Source: CAD feature listing. Evaluate the final solid. Frame: model axes, mm. A direction names the side the tool comes from. Coordinates: 2 decimals unless noted, no trailing zeros. Order: outer loops, then holes, each group sorted by start corner. A loop starts at its lowest first (then second) coordinate and runs counter-clockwise, first axis right, second up.
Item 1: Section C-C on x = 4. Return the cut outline in (y, z), then the cut area to 3 significant figures.
Item 2: Reachability of faces 1 (the flat face through (80.5, 0, 8.2)), 2 (the flat face through (82.5, 0, 0)) from +Z, -Z, +X, -X, +Y, -Y: full face, straight path, thin tool, end or side. Return the list, or none.
Item 3: Section A-A on y = 0. Return the cut outline in (x, z).
Item 4: Ray query, line 1 (X direction, y = 0, z = -3.75); line 2 (X direction, y = -1.25, z = 9.25); line 3 (Y direction, x = 4, z = -5.25). Return the intervals inside material, ascending.
Item 5: Contact query for flat-ended pins moving along their axis: P1, Ø1, axis at x = 52.5, y = -2, coming from the +Z side; P2, Ø1, axis at x = 30.5, y = -6, coming from the +Z side; P3, Ø6, axis at x = 45.5, z = -3.5, coming from the +Y side; P4, Ø8, axis at y = 7, z = 7.5, coming from the -X side. Output: stop coordinate, or through.
Item 6: Section B-B on x = 60. Return the cut outline in (y, z), then the cut area to 3 significant figures.
from build123d import *

# Parameters (mm, degrees)
SCHNITT_LINEAR_AUSTRAGEN1_REACH             = 12
SKIZZE2_R                                   = 1
SCHNITT_LINEAR_AUSTRAGEN1_DIRECTION_2_DEPTH = 11
VERRUNDUNG1_R                               = 1


with BuildPart() as part:
    # Skizze1 → Rotation1 (revolve)
    with BuildSketch(Plane.XY):
        Polygon((0, 0), (0, 8), (80.5, 8), (80.5, 10), (82.5, 10), (82.5, 0), align=None)
    revolve(axis=Axis((-15.956588212, 0, 0), (1, 0, 0)))

    # Skizze2 → Schnitt-Linear austragen1 (cut, up to next)
    with BuildSketch(Plane.XY, mode=Mode.PRIVATE) as schnitt_linear_austragen1_sk1:
        with Locations((4, 0)):
            Circle(SKIZZE2_R)
    schnitt_linear_austragen1_tool1 = extrude(schnitt_linear_austragen1_sk1.sketch, amount=-SCHNITT_LINEAR_AUSTRAGEN1_REACH, mode=Mode.PRIVATE) & part.part
    add(schnitt_linear_austragen1_tool1.solids().sort_by_distance((4, 0, 0))[0], mode=Mode.SUBTRACT)

    # Skizze2 → Schnitt-Linear austragen1 direction 2 (cut)
    with BuildSketch(Plane.XY):
        with Locations((4, 0)):
            Circle(SKIZZE2_R)
    extrude(amount=SCHNITT_LINEAR_AUSTRAGEN1_DIRECTION_2_DEPTH, mode=Mode.SUBTRACT)

    # Verrundung1
    verrundung1_edges = [part.edges().sort_by_distance(p)[0] for p in [
        (0, -8, 0),
    ]]
    fillet(verrundung1_edges, radius=VERRUNDUNG1_R)


solid = part.part
Answer list:
1. outline: (-1, -7.94) - (-1, 7.94) arc R8 ccw to start; (1, -7.94) arc R8 ccw to (1, 7.94) - close
1. area: 169 mm2
2. face 1: -X
2. face 2: +Z, -Z, +X, +Y, -Y
3. outline: (0, -7) arc R1 ccw to (1, -8) - (3, -8) - (3, 8) - (1, 8) arc R1 ccw to (0, 7) - close; (5, -8) - (80.5, -8) - (80.5, -10) - (82.5, -10) - (82.5, 10) - (80.5, 10) - (80.5, 8) - (5, 8) - close
4. line 1: x = 0 to 3, 5 to 82.5
4. line 2: x = 80.5 to 82.5
4. line 3: y = -6.04 to -1, 1 to 6.04
5. P1: stops at z = 7.86
5. P2: stops at z = 5.81
5. P3: stops at y = 7.98
5. P4: stops at x = 0
6. outline: circle Ø16 at (0, 0)
6. area: 201 mm2
